The figure shows three views and two pictorial views of one solid part (mm, origin at its lowest corner). Answer the questions. Coordinates: 2 decimals unless noted, no trailing zeros. Loops run counter-clockwise (first coordinate to the right, second up) from the corner with the lowest first, then second, coordinate; pieces in that order, holes last. Notation, with made-up numbers: (85, -2.75) - (121, -2.75) arc R10 ccw to (121, 13.25) - close; hole circle Ø5 at (57, 59). An arc over 180 degrees is marked (long way). One line per question, with ' | ' between items.
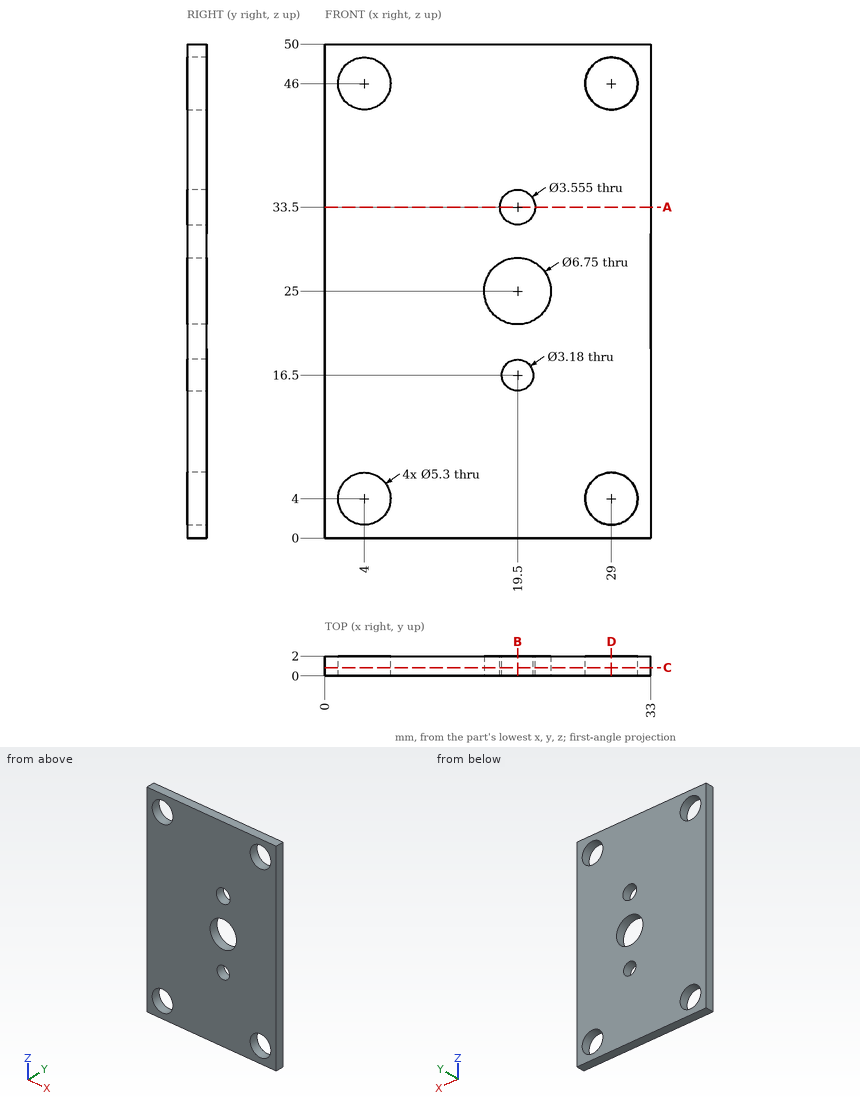
Item 1: Find section B-B, the plane x = 19.5. Write down the section's boundary in (y, z) (1 decimal).
Taken from the geometry:
outline: (0, 0) - (2, 0) - (2, 14.9) - (0, 14.9) - close; (0, 18.1) - (2, 18.1) - (2, 21.6) - (0, 21.6) - close; (0, 28.4) - (2, 28.4) - (2, 31.7) - (0, 31.7) - close; (0, 35.3) - (2, 35.3) - (2, 50) - (0, 50) - close
Item 2: Find section C-C, the plane y = 0.85. State how many separate pieces and enclosed holes the cut face has, plus the area to 3 significant figures.
Taken from the geometry:
separate pieces: 1 | enclosed holes: 7 | area: 1,510 mm2
Item 3: Find section D-D, the plane x = 29. Write down the section's boundary in (y, z).
Taken from the geometry:
outline: (0, 0) - (2, 0) - (2, 1.35) - (0, 1.35) - close; (0, 6.65) - (2, 6.65) - (2, 43.35) - (0, 43.35) - close; (0, 48.65) - (2, 48.65) - (2, 50) - (0, 50) - close
Item 4: Find the intervals of material crossed by line 1 (Z direction, x = 29, y = 1); line 2 (X direction, y = 0.6, z = 4); line 3 (Z direction, x = 18.5, y = 1.4) (1 decimal), in increasing order. Write a range as [from, to].
Taken from the geometry:
line 1: z = [0, 1.35], [6.65, 43.35], [48.65, 50] | line 2: x = [0, 1.35], [6.65, 26.35], [31.65, 33] | line 3: z = [0, 15.3], [17.7, 21.8], [28.2, 32], [35, 50]
Item 5: This flat-tipped pin is pushed along its axis until it touches: pin 1 Ø3 at (x, z) = (4, 4) entering from -Y (3 decimals). Where does it stop, or does it pass through?
Taken from the geometry:
pin 1: passes through
Item 6: Find section A-A, the plane z = 33.5. Write down the section's boundary in (x, y).
Taken from the geometry:
outline: (0, 0) - (17.72, 0) - (17.72, 2) - (0, 2) - close; (21.28, 0) - (33, 0) - (33, 2) - (21.28, 2) - close
